The model under review builds one solid part; all positions refer to its coordinate system, in mm. Face numbers are marked on the shaded views. Give positions to 0.01 mm unless a question says otherwise; leave off trailing zeros. Loops run counter-clockwise (first coordinate to the right, second up) from the corner with the lowest first, then second, coordinate; pieces in that order, holes last. Notation, with made-up numbers: (-2.5, -30) - (20.5, -30) arc R18 ccw to (20.5, -16) - close; hole circle Ø4 at (36.5, -32.75). An arc over 180 degrees is marked (long way). Answer as a JSON object with one key per item and string values.
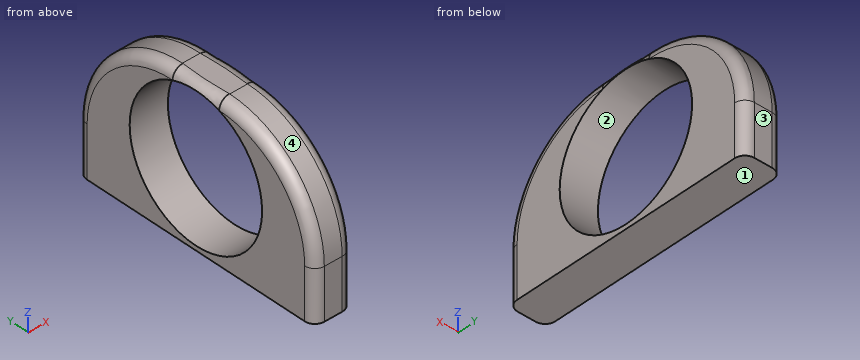
Autodesk Fusion 360 part; units mm, degrees
sketch "Sketch1" plane through (0, 0, 0) normal (0, 0, 1) x (1, 0, 0)
  line L0 (0.9525, 6.35) -> (-0.9525, 6.35)
  line L1 (-0.9525, 6.35) -> (-0.9525, -6.35)
  line L2 (-0.9525, -6.35) -> (0.9525, -6.35)
  line L3 (0.9525, -6.35) -> (0.9525, 6.35)
  line L4 (0.9525, 6.35) -> (-0.9525, -6.35) construction
  line L5 (-0.9525, 6.35) -> (0.9525, -6.35) construction
  dimension "d7" = 1.905
  dimension "d8" = 12.7
extrude "Extrude1" add sketch "Sketch1" along normal blind 7.62
sketch "Sketch2" plane through (0.9525, 0, 0) normal (1, 0, 0) x (0, 0, -1)
  line L0 (0, -6.35) -> (0, 6.35)
  line L1 (0, 6.35) -> (-7.62, 6.35)
  line L2 (-7.62, 6.35) -> (-7.62, -6.35)
  line L3 (-7.62, -6.35) -> (0, -6.35)
  circle A0 centre (-3.7773, 0) radius 3.556
  dimension "d11" = 7.112
extrude "Extrude2" cut sketch "Sketch2" against normal blind 12.7 contours A0
sketch "Sketch3" plane through (0, 0, 0) normal (0, 0, -1) x (-1, 0, 0)
  line L0 (-0.9525, 6.35) -> (-0.9525, -6.35)
  line L1 (-0.9525, -6.35) -> (0.9525, -6.35)
  line L2 (0.9525, -6.35) -> (0.9525, 6.35)
  line L3 (0.9525, 6.35) -> (-0.9525, 6.35)
  point P0 (-0.9525, 0)
fillet "Fillet1" radius 5.08 2 edges at (0, 6.35, 7.62) (0, -6.35, 7.62)
fillet "Fillet2" radius 0.508 10 edges at (0.9525, -6.35, 1.27) (0.9525, -4.8621, 6.1321) (0.9525, 0, 7.62) (0.9525, 4.8621, 6.1321) (0.9525, 6.35, 1.27) (-0.9525, 6.35, 1.27) (-0.9525, 4.8621, 6.1321) (-0.9525, 0, 7.62) (-0.9525, -4.8621, 6.1321) (-0.9525, -6.35, 1.27)
equation "tabHeight = 0.3 in"
equation "tabWidth = 0.5 in"
equation "tabThickness = 0.075 in"
equation "pinSize = 0.25 in"
equation "pinHoleClearance = 0.03 in"
equation "pinHoleDiameter = pinSize + pinHoleClearance"
equation "d7 = tabThickness"
equation "d8 = tabWidth"
equation "d9 = tabHeight"
equation "d11 = pinHoleDiameter"
Q1. Clearance check with flat-ended pins moving along their axes: pin 1 Ø1 at (x, z) = (0, 4.5) entering from +Y; pin 2 Ø4.5 at (y, z) = (0, 3.78) entering from +X. State where each tip first meets the part, or that it passes through.
Results:
{"pin 1": "stops at y = 6.14", "pin 2": "passes through"}
Q2. Consider section A-A, the plane x = -0.1. State the section outline as (y, z) points, plus the area to 3 significant figures.
Results:
{"outline": "(-6.35, 0) - (6.35, 0) - (6.35, 2.54) arc R5.08 ccw to (1.27, 7.62) - (-1.27, 7.62) arc R5.08 ccw to (-6.35, 2.54) - close; hole circle Ø7.11 at (0, 3.78)", "area": "46.0 mm^2"}
Q3. To check wall thickness, follow probe 1 along Z at (x, y) = (0.35, 0); probe 2 along Z at (x, y) = (0.45, 2.5); probe 3 along Y at (x, z) = (-0.3, 3.5). State the ranges of each line that lie inside material, in increasing order. Write a range as [from, to].
Results:
{"probe 1": "z = [0, 0.22], [7.33, 7.62]", "probe 2": "z = [0, 1.25], [6.31, 7.47]", "probe 3": "y = [-6.26, -3.55], [3.55, 6.26]"}
Q4. Consider section B-B, the plane z = 0.75. State the section outline as (x, y) points.
Results:
{"outline": "(-0.95, -5.84) arc R0.51 ccw to (-0.44, -6.35) - (0.44, -6.35) arc R0.51 ccw to (0.95, -5.84) - (0.95, -1.87) - (-0.95, -1.87) - close; (-0.95, 1.87) - (0.95, 1.87) - (0.95, 5.84) arc R0.51 ccw to (0.44, 6.35) - (-0.44, 6.35) arc R0.51 ccw to (-0.95, 5.84) - close"}
Q5. The part is to be moulded in two halves that separate along Z. For the marked faces 1, 2, 3 and 4, say which applies: +Z half, -Z half, draft (parallel to the pull), parting line (faces both ways), or undercut.
Results:
{"face 1": "-Z half", "face 2": "undercut", "face 3": "draft", "face 4": "+Z half"}
